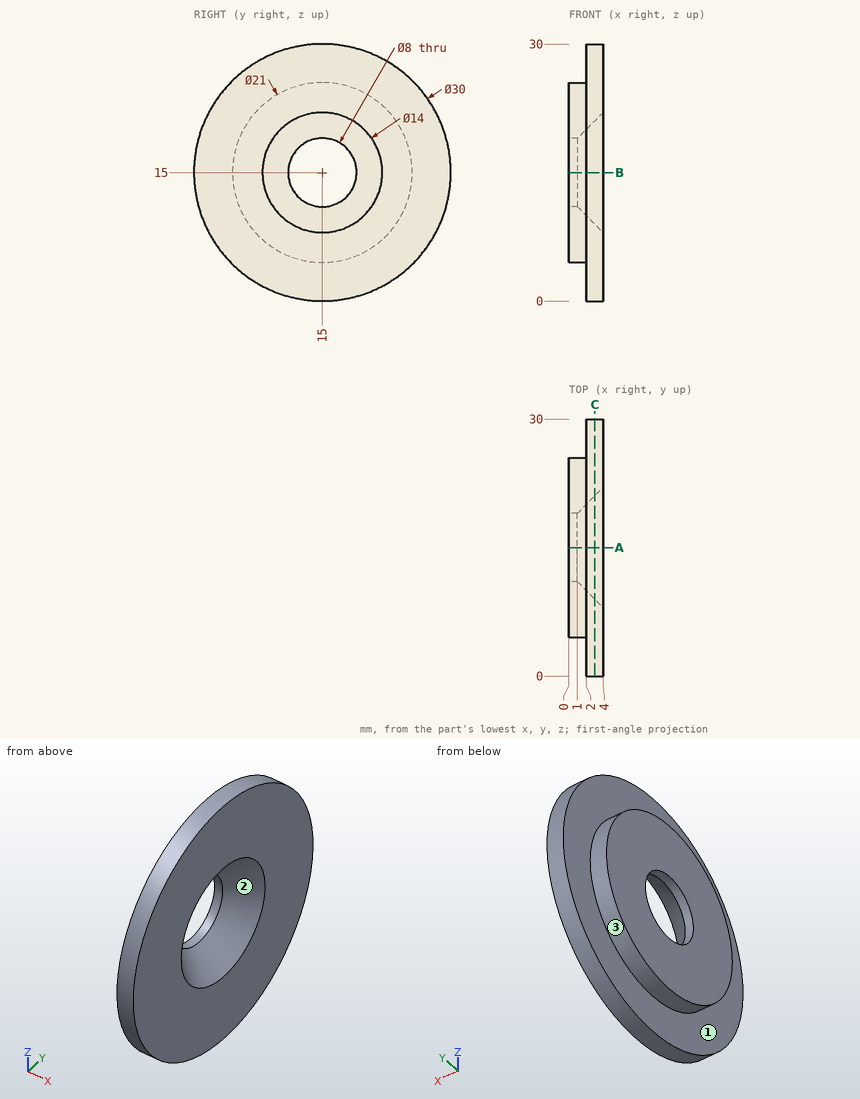
Verification items for this drawing (mm, ordinates from the low corner). Coordinates: 2 decimals unless noted, no trailing zeros. Order: outer loops, then holes, each group sorted by start corner. A loop starts at its lowest first (then second) coordinate and runs counter-clockwise, first axis right, second up. Notation, with made-up numbers: (-40, 49) -> (0, 49) arc R18 cw to (0, 84) -> close; hole circle Ø3 at (73.25, 1.5). An arc over 180 degrees is marked (long way). Put each result on its own line as item: value. Start each with the question number.
1. Material ranges on L1, parallel to Y at x = 0.2, z = 15; L2, parallel to Y at x = 2.35, z = 11.75, recorded low to high. Write a range as [from, to].
2. Cross-section at C-C, the plane x = 3.05. Record the boundary of the cut face in (y, z), then the cut area to 3 significant figures.
3. Cross-section at A-A, the plane y = 15. Record the boundary of the cut face in (x, z), then the cut area to 3 significant figures.
4. Go/stop test with flat-tipped pins: pin 1 Ø12 at (y, z) = (20.5, 5.5) entering from -X; pin 2 Ø1.5 at (x, y) = (2.5, 17.5) entering from +Z; pin 3 Ø1.5 at (x, z) = (2.5, 26) entering from -Y; pin 4 Ø1.5 at (x, z) = (2, 11) entering from +Y. Record where each tip stops, or that it passes through.
5. Mould release check, pull along Z, two halves, no side actions. Record for the marked faces 1, 2 and 3: released by +Z, released by -Z, zero draft, split by the parting line, or undercut.
Computed:
1. L1: [4.5, 11], [19, 25.5]
1. L2: [0.36, 10.75], [19.25, 29.64]
2. outline: circle Ø30 at (15, 15); hole circle Ø12.1 at (15, 15)
2. area: 592 mm2
3. outline: (0, 4.5) -> (2, 4.5) -> (2, 0) -> (4, 0) -> (4, 8) -> (1, 11) -> (0, 11) -> close; (0, 19) -> (1, 19) -> (4, 22) -> (4, 30) -> (2, 30) -> (2, 25.5) -> (0, 25.5) -> close
3. area: 61.0 mm2
4. pin 1: x = 0
4. pin 2: z = 29.9
4. pin 3: y = 4.05
4. pin 4: y = 29.64
5. face 1: zero draft
5. face 2: undercut
5. face 3: split by the parting line
